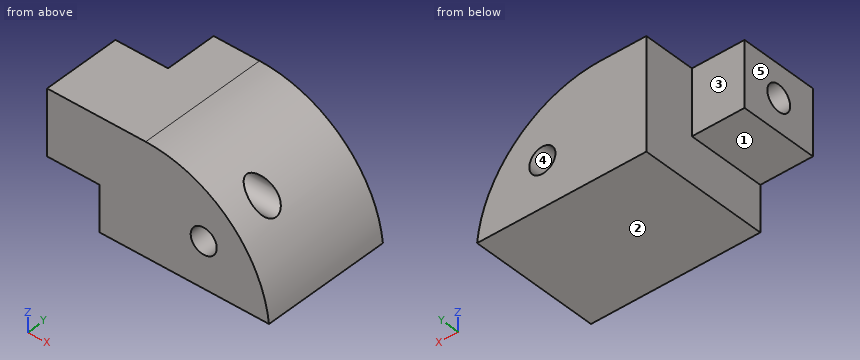
```python
from build123d import *

# Parameters (mm, degrees)
F0_W        = 215.9
F0_H        = 127
F1_DEPTH    = 107.95
F4_W        = 50.8
F4_H        = 50.8
F5_DEPTH    = 107.95
F6_DEPTH    = 51.21156
F7_T1_DEPTH = 726.8985851792
F9_D        = 25.4
F10_D       = 25.4


# Not quite as in the source:
# - a fillet or chamfer that OpenCascade refuses, or shapes differently, is made with other operations: its cross-section is extruded or revolved along the edge and cut away or added


with BuildPart() as f1:
    # F0 (on Top) → F1 (new body)
    with BuildSketch(Plane.XY):
        with Locations((-26.1275832451, 6.2899636105)):
            Rectangle(F0_W, F0_H)
    extrude(amount=F1_DEPTH)

    # F4 (on face) → F5 (cut)
    with BuildSketch(Plane.XY.offset(107.95)):
        with Locations((-108.6775832451, 44.3899636105)):
            Rectangle(F4_W, F4_H)
    extrude(amount=-F5_DEPTH, mode=Mode.SUBTRACT)

    # F2 (on face) → F6 (cut)
    with BuildSketch(Plane(origin=(-134.0775832451, 0, 0), x_dir=(0, -1, 0), z_dir=(-1, 0, 0))):
        Polygon((-18.9899636105, 44.45), (-18.9899636105, 107.95), (-69.7899636105, 107.95), (-69.7899636105, 0), (57.2100363895, 0), (57.2100363895, 44.45), align=None)
    extrude(amount=-F6_DEPTH, mode=Mode.SUBTRACT)

    # F7: fillet of radius 120.65 on 1 edges, made by hand

    # F7_s2 → F7_t1 (cut)
    with BuildSketch(Plane.XZ.offset(-369.7392562001)):
        with BuildLine():
            ThreePointArc((81.8224167549, 0), (42.5401826414, 76.9902377631), (-38.1573002809, 107.95))
            Line((-38.1573002809, 107.95), (81.8224167549, 107.95))
            Line((81.8224167549, 107.95), (81.8224167549, 0))
        make_face()
    extrude(amount=F7_T1_DEPTH, mode=Mode.SUBTRACT)

    # F9 (through all)
    with Locations(Plane.XZ.offset(57.2100363895)):
        with Locations((18.3224167549, 44.45)):
            Hole(F9_D / 2)

    # F10 (through all)
    with Locations(Plane(origin=(-134.0775832451, 0, 0), x_dir=(0, -1, 0), z_dir=(-1, 0, 0))):
        with Locations((19.1100363895, 76.2)):
            Hole(F10_D / 2)


solid = f1.part
```
Check sheet for the modelled part. Datum: model origin and axes. Units: mm. Face numbers are marked on the shaded views. A direction names the side the tool comes from. Round coordinates to 2 decimals unless told otherwise and drop trailing zeros. Loops run counter-clockwise (first coordinate to the right, second up) from the corner with the lowest first, then second, coordinate; pieces in that order, holes last. Notation, with made-up numbers: (35, 43.25) - (88, 43.25) arc R22 cw to (88, 54.25) - close; hole circle Ø1 at (21.25, 27.5). An arc over 180 degrees is marked (long way). Write item = value, one per line. Start each with the question number.
Q1. Section check B-B (y = -13). Record the boundary of the cut face in (x, z), plus the area to 3 significant figures.
Q2. Section check A-A (y = 5.5). Record the boundary of the cut face in (x, z), plus the area to 3 significant figures.
Q3. Release check for a two-part mould opening along X. For the marked faces 3, 4 and 5 record: pulls with the +X half, pulls with the -X half, needs draft (parallel to the pull), parting line crosses it, or undercut.
Q4. Section check D-D (z = 76.2). Record the boundary of the cut face in (x, y), plus the area to 3 significant figures.
Q5. Depth check by flat-ended pin: P1, Ø5, axis at y = 52.5, z = 97, coming from the +X side; P2, Ø12, axis at x = -89.5, y = 27, coming from the +Z side; P3, Ø3, axis at x = -64, y = 44.5, coming from the -Z side; P4, Ø3, axis at y = 40, z = 26.5, coming from the +X side. Enter the tip coordinate at first touch or a pass-through.
Q6. Thickness scan on L1, parallel to Z at x = 25.5, y = -28; L2, parallel to Y at x = -29, z = 76.2; L3, parallel to X at y = 32, z = 44. Record the ranges inside material, lowest first.
Q7. Section check C-C (x = -99). Record the boundary of the cut face in (y, z).
Q8. Access from +Z, -Z, +X, -X, +Y, -Y to the whole of each face (thin tool, end or side, straight path). Record for the marked faces 1 and 2.
Derived:
q1.outline = (-134.08, 44.45) - (-82.87, 44.45) - (-82.87, 0) - (81.82, 0) arc R120.65 ccw to (54.09, 65.07) - (-134.08, 65.07) - close; (-134.08, 87.33) - (29.29, 87.33) arc R120.65 ccw to (-38.16, 107.95) - (-134.08, 107.95) - close; hole circle Ø25.4 at (18.32, 44.45)
q1.area = 13,500 mm^2
q2.outline = (-134.08, 44.45) - (-82.87, 44.45) - (-82.87, 0) - (81.82, 0) arc R120.65 ccw to (-38.16, 107.95) - (-134.08, 107.95) - close; hole circle Ø25.4 at (18.32, 44.45)
q2.area = 17,500 mm^2
q3.face_3 = needs draft
q3.face_4 = undercut
q3.face_5 = pulls with the -X half
q4.outline = (-134.08, -57.21) - (43.41, -57.21) - (43.41, -31.81) - (-134.08, -31.81) - close; (-134.08, -6.41) - (43.41, -6.41) - (43.41, 69.79) - (-82.87, 69.79) - (-82.87, 18.99) - (-134.08, 18.99) - close
q4.area = 15,400 mm^2
q5.P1 = 17.2
q5.P2 = through
q5.P3 = 0
q5.P4 = 76.45
q6.L1 = 0 to 33.97, 54.93 to 67.13, 85.27 to 89.79
q6.L2 = -57.21 to -31.81, -6.41 to 69.79
q6.L3 = -82.87 to 5.63, 31.01 to 68.34
q7.outline = (-57.21, 44.45) - (18.99, 44.45) - (18.99, 107.95) - (-57.21, 107.95) - close; hole circle Ø25.4 at (-19.11, 76.2)
q8.face_1 = -Z, -X, +Y, -Y
q8.face_2 = -Z, +X, -X, +Y, -Y
